```python
from build123d import *

# Parameters (mm, degrees)
TAP_DRILL_FOR_M3X0_5_TAP1_D     = 2.5
TAP_DRILL_FOR_M3X0_5_TAP1_DEPTH = 5
TAP_DRILL_FOR_M3X0_5_TAP1_TIP   = 0.751075774


with BuildPart() as part:
    # Sketch1 → Revolve1 (revolve)
    with BuildSketch(Plane(origin=(0, 0, 0), x_dir=(0, 0, -1), z_dir=(1, 0, 0)), mode=Mode.PRIVATE) as revolve1_sk:
        Polygon((0, 0), (0, -2), (-10, -2), (-10, -3.5), (-13, -3.5), (-13, -12.5), (-61, -12.5), (-61, 0), align=None)
    revolve(revolve1_sk.sketch.rotate(Axis((0, 0, 61), (0, 0, -1)), 270), axis=Axis((0, 0, 61), (0, 0, -1)))

    # Tap Drill for M3x0.5 Tap1
    with Locations(Plane(origin=(0, 0, 13), x_dir=(-1, 0, 0), z_dir=(0, 0, -1))):
        with Locations((-8.5, 0), (8.5, 0)):
            Hole(TAP_DRILL_FOR_M3X0_5_TAP1_D / 2, depth=TAP_DRILL_FOR_M3X0_5_TAP1_DEPTH)
            with Locations((0, 0, -(TAP_DRILL_FOR_M3X0_5_TAP1_DEPTH + TAP_DRILL_FOR_M3X0_5_TAP1_TIP / 2))):  # 118° drill point
                Cone(0, TAP_DRILL_FOR_M3X0_5_TAP1_D / 2, TAP_DRILL_FOR_M3X0_5_TAP1_TIP, mode=Mode.SUBTRACT)


solid = part.part
```
Geometry: final body of the model. Coordinates: model frame, mm. A direction names the side the tool comes from. Coordinates: 2 decimals unless noted, no trailing zeros. Loops run counter-clockwise (first coordinate to the right, second up) from the corner with the lowest first, then second, coordinate; pieces in that order, holes last. Notation, with made-up numbers: (39, 15) -> (61, 15) arc R15 cw to (61, 19) -> close; hole circle Ø9 at (-3.75, -39.5). An arc over 180 degrees is marked (long way). Use a Markdown table: item, result. Add a question column.
(1) Section query C-C, the plane y = -7.5. Return loops of the section in (x, z).
(2) Pin query (flat end, axial travel): pin 1 Ø1 at (x, z) = (6, 43) entering from +Y (3 decimals); pin 2 Ø2 at (x, z) = (-2.5, 40) entering from -Y; pin 3 Ø1.5 at (y, z) = (8.5, 42) entering from +X. Return the tip coordinate at first contact, or that it passes through.
(3) Access query for faces 4 (the flat face through (0, 0, 0)), 5 (the flat face through (-3, 3, 13)). Directions: +Z, -Z, +X, -X, +Y, -Y. A direction counts if a zero-diameter tool reaches every point of the face in a straight line with its end or side. Return the directions, or none.
(4) Section query A-A, the plane x = 0. Return loops of the section in (y, z), plus the area to 3 significant figures.
(5) Section query D-D, the plane z = 42. Return loops of the section in (x, y).
(6) Mould query, pull axis Y, two halves, no side actions, for faces 1 (the cylindrical face through (-9.75, 0.05, 15.54)), 2 (the flat face through (-2, 2, 10)), 3 (the cylindrical face through (11.923, -3.755, 37.336)). Classes: pulls with the +Y half, pulls with the -Y half, needs draft (parallel to the pull), parting line crosses it, or undercut.
(7) Line query: line 1 along Z through (x, y) = (4.5, -8); line 2 along Y through (x, z) = (8.5, 14.65); line 3 along Y through (x, z) = (0.25, 51.5). Output: solid intervals per line, ascending.
(8) Section query B-B, the plane z = 8.5. Return loops of the section in (x, y).
Answer:
| question | item | result |
|---|---|---|
| 1 | outline | (-10, 13) -> (10, 13) -> (10, 61) -> (-10, 61) -> close |
| 2 | pin 1 | stops at y = 11.225 |
| 2 | pin 2 | stops at y = -12.41 |
| 2 | pin 3 | stops at x = 9.81 |
| 3 | face 4 | -Z, +X, -X, +Y, -Y |
| 3 | face 5 | -Z |
| 4 | outline | (-12.5, 13) -> (-3.5, 13) -> (-3.5, 10) -> (-2, 10) -> (-2, 0) -> (2, 0) -> (2, 10) -> (3.5, 10) -> (3.5, 13) -> (12.5, 13) -> (12.5, 61) -> (-12.5, 61) -> close |
| 4 | area | 1,260 mm^2 |
| 5 | outline | circle Ø25 at (0, 0) |
| 6 | face 1 | undercut |
| 6 | face 2 | needs draft |
| 6 | face 3 | parting line crosses it |
| 7 | line 1 | z = 13 to 61 |
| 7 | line 2 | y = -9.17 to -1.25, 1.25 to 9.17 |
| 7 | line 3 | y = -12.5 to 12.5 |
| 8 | outline | circle Ø4 at (0, 0) |
